Geometry: final body of the model. Coordinates: model frame, mm. Coordinates: 2 decimals unless noted, no trailing zeros. Order: outer loops, then holes, each group sorted by start corner. A loop starts at its lowest first (then second) coordinate and runs counter-clockwise, first axis right, second up. Notation, with made-up numbers: M 81,-37.75 L 118,-37.75 A23 cw 118,-11.75 Z; hole C 83,65.25 d10. An arc over 180 degrees is marked long. Write item = value, one per line. Start each with the question number.
```python
from build123d import *

# Parameters (mm, degrees)
SKETCH1_R             = 3
BOSS_EXTRUDE1_DEPTH   = 10
M3X0_5_TAPPED_HOLE1_D = 2.5
CHAMFER1_SIZE         = 0.5


with BuildPart() as part:
    # Sketch1 → Boss-Extrude1 (new body)
    with BuildSketch(Plane(origin=(0, 0, 0), x_dir=(1, 0, 0), z_dir=(0, 1, 0))):
        with Locations(Location((0, 0, 0), (0, 0, 270))):
            Circle(SKETCH1_R)
    extrude(amount=BOSS_EXTRUDE1_DEPTH)

    # M3x0.5 Tapped Hole1 (through all)
    with Locations(Plane(origin=(0, 10, 0), x_dir=(1, 0, 0), z_dir=(0, 1, 0))):
        with Locations((0, 0)):
            Hole(M3X0_5_TAPPED_HOLE1_D / 2)

    # Chamfer1
    chamfer1_edges = [part.edges().sort_by_distance(p)[0] for p in [
        (0, 0, -3),
        (0, 10, -3),
    ]]
    chamfer(chamfer1_edges, length=CHAMFER1_SIZE)


solid = part.part
```
Item 1: Section query C-C on y = 5.25. Output: boundary loops of the cut face in (x, z), and give its area (3 significant figures).
Item 2: Material intervals for probe 1 along Z at (x, y) = (0.2, 7); probe 2 along X at (y, z) = (6, -0.55); probe 3 along Z at (x, y) = (1.4, 3.25), sorted ascending. Write a range as [from, to].
Item 3: First-contact query: pin 1 (3 mm diameter, centred on y = 4.5, z = 2, fed in from -X); pin 2 (1.5 mm diameter, centred on x = 0, z = 0, fed in from +Y). Flat tips, straight axial feed; report the tip coordinate or a pass-through.
Item 4: Section query B-B on x = 0. Output: boundary loops of the cut face in (y, z).
Item 5: Section query A-A on z = 0. Output: boundary loops of the cut face in (x, y).
Item 6: Draft query along Z for faces 1 (the cylindrical face through (0.9, 4.94, 2.86)), 2 (the cylindrical face through (0.27, 4.93, 1.22)), 3 (the flat face through (1, 0, 1)). Return one class per face: pulls with the +Z half, pulls with the -Z half, needs draft (parallel to the pull), parting line crosses it, or undercut.
Ans:
q1.outline = C 0,0 d6; hole C 0,0 d2.5
q1.area = 23.4 mm^2
q2.probe_1 = [-2.99, -1.23], [1.23, 2.99]
q2.probe_2 = [-2.95, -1.12], [1.12, 2.95]
q2.probe_3 = [-2.65, 2.65]
q3.pin_1 = -2.96
q3.pin_2 = through
q4.outline = M 0,-2.5 L 0.5,-3 L 9.5,-3 L 10,-2.5 L 10,-1.25 L 0,-1.25 Z; M 0,1.25 L 10,1.25 L 10,2.5 L 9.5,3 L 0.5,3 L 0,2.5 Z
q5.outline = M -3,0.5 L -2.5,0 L -1.25,0 L -1.25,10 L -2.5,10 L -3,9.5 Z; M 1.25,0 L 2.5,0 L 3,0.5 L 3,9.5 L 2.5,10 L 1.25,10 Z
q6.face_1 = parting line crosses it
q6.face_2 = undercut
q6.face_3 = needs draft
